Geometry check sheet. Reference: the model listing, model coordinates, mm. A direction names the side the tool comes from. Give positions to 0.01 mm unless a question says otherwise; leave off trailing zeros. Order: outer loops, then holes, each group sorted by start corner. A loop starts at its lowest first (then second) coordinate and runs counter-clockwise, first axis right, second up.
Autodesk Inventor part; units mm, degrees
ref_plane "YZ Plane" through (0, 0, 0) normal (1, 0, 0) x (0, 1, 0)
ref_plane "XZ Plane" through (0, 0, 0) normal (0, 1, 0) x (-1, 0, 0)
ref_plane "XY Plane" through (0, 0, 0) normal (0, 0, 1) x (1, 0, 0)
sketch "Sketch1" plane through (0, 0, 0) normal (0, 1, 0) x (-1, 0, 0)
  circle A0 centre (0, 0) radius 4
  circle A1 centre (0, 0) radius 11
  dimension "d0" = 8
  dimension "d1" = 22
extrude "Extrusion1" add sketch "Sketch1" along normal blind 7
sketch "Sketch2" plane through (0, 7, 0) normal (0, 1, 0) x (1, 0, 0)
  circle A0 centre (0, 0) radius 4
  circle A1 centre (0, 0) radius 11
  circle A2 centre (0, 0) radius 9
  circle A3 centre (0, 0) radius 6
  dimension "d4" = 2
  dimension "d5" = 2
extrude "Extrusion2" cut sketch "Sketch2" against normal blind 0.1 contours A2
sketch "Sketch3" plane through (0, 0, 0) normal (0, -1, 0) x (1, 0, 0)
  circle A0 centre (0, 0) radius 4
  circle A1 centre (0, 0) radius 11
  circle A2 centre (0, 0) radius 9
  circle A3 centre (0, 0) radius 6
extrude "Extrusion3" cut sketch "Sketch3" against normal blind 0.1 contours A2
properties part number "608 skate bearing"
Q1. Release check for a two-part mould opening along X. For faces 1 (the face through (2.38, 3.45, 10.74)), 2 (the face through (2, 0.1, -6)), 3 (the face through (1.42, 7, -3.92)) record: pulls with the +X half, pulls with the -X half, needs draft (parallel to the pull), parting line crosses it, or undercut.
Q2. Gauge pin test, flat ends, axial feed: P1, Ø5.5, axis at x = -2, z = 1.5, coming from the +Y side; P2, Ø1.5, axis at x = -6.5, y = 1, coming from the -Z side; P3, Ø1.5, axis at y = 6, z = -7.5, coming from the +X side; P4, Ø4, axis at x = 2.5, y = 5, coming from the +Z side. Record the tip position at first contact, or that the pin passes through.
Q3. Cross-section at C-C, the plane y = 3. Record the boundary of the cut face in (x, z).
Q4. Thickness scan on L1, parallel to Z at x = 0, y = 4.75; L2, parallel to Y at x = 6, z = -4; L3, parallel to Z at x = 1, y = 2. Record the ranges inside material, lowest first.
Q5. Cross-section at A-A, the plane z = 0. Record the boundary of the cut face in (x, y), and give its area (3 significant figures).
Q6. Cross-section at D-D, the plane x = 4.5. Record the boundary of the cut face in (y, z), and give its area (3 significant figures).
Q7. Access from +Z, -Z, +X, -X, +Y, -Y to the whole of each face (thin tool, end or side, straight path). Record for faces 4 (the face through (2, 6.9, 6)), 5 (the face through (0.867, 3.451, 3.905)).
Q8. Cross-section at B-B, the plane x = 0. Record the boundary of the cut face in (y, z), and give its area (3 significant figures).
Answers follow:
1. face 1: parting line crosses it
1. face 2: undercut
1. face 3: needs draft
2. P1: stops at y = 7
2. P2: stops at z = -9.38
2. P3: stops at x = 8.69
2. P4: stops at z = 10.99
3. outline: circle Ø22 at (0, 0); hole circle Ø8 at (0, 0)
4. L1: z = -11 to -4, 4 to 11
4. L2: y = 0.1 to 6.9
4. L3: z = -10.95 to -3.87, 3.87 to 10.95
5. outline: (-11, 0) - (-9, 0) - (-9, 0.1) - (-6, 0.1) - (-6, 0) - (-4, 0) - (-4, 7) - (-6, 7) - (-6, 6.9) - (-9, 6.9) - (-9, 7) - (-11, 7) - close; (4, 0) - (6, 0) - (6, 0.1) - (9, 0.1) - (9, 0) - (11, 0) - (11, 7) - (9, 7) - (9, 6.9) - (6, 6.9) - (6, 7) - (4, 7) - close
5. area: 96.8 mm2
6. outline: (0, -10.04) - (7, -10.04) - (7, -7.79) - (6.9, -7.79) - (6.9, -3.97) - (7, -3.97) - (7, 3.97) - (6.9, 3.97) - (6.9, 7.79) - (7, 7.79) - (7, 10.04) - (0, 10.04) - (0, 7.79) - (0.1, 7.79) - (0.1, 3.97) - (0, 3.97) - (0, -3.97) - (0.1, -3.97) - (0.1, -7.79) - (0, -7.79) - close
6. area: 139 mm2
7. face 4: +Y
7. face 5: +Y, -Y
8. outline: (0, -11) - (7, -11) - (7, -9) - (6.9, -9) - (6.9, -6) - (7, -6) - (7, -4) - (0, -4) - (0, -6) - (0.1, -6) - (0.1, -9) - (0, -9) - close; (0, 4) - (7, 4) - (7, 6) - (6.9, 6) - (6.9, 9) - (7, 9) - (7, 11) - (0, 11) - (0, 9) - (0.1, 9) - (0.1, 6) - (0, 6) - close
8. area: 96.8 mm2
